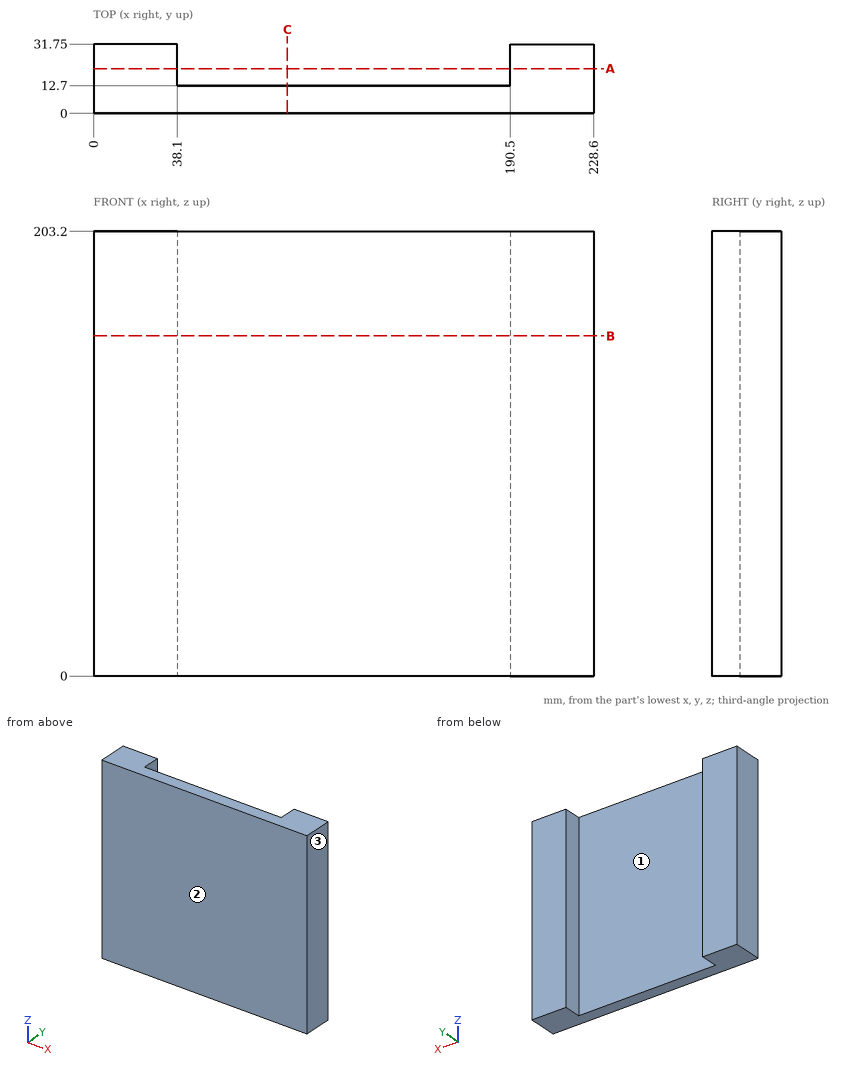
Input: dimensioned drawing with shaded views. Units: mm. Origin: part minimum x, y, z. Coordinates: 2 decimals unless noted, no trailing zeros. Order: outer loops, then holes, each group sorted by start corner. A loop starts at its lowest first (then second) coordinate and runs counter-clockwise, first axis right, second up. Notation, with made-up numbers: (55.5, -14) - (87.5, -14) arc R3 cw to (87.5, -10) - close; hole circle Ø8 at (75.5, 74). An arc over 180 degrees is marked (long way). Return JSON: item names as keys, results as strings. Group by question number.
1. Cut plane B-B (z = 155.5). Output: boundary loops of the cut face in (x, y), plus the area to 3 significant figures.
2. Cut plane C-C (x = 88.5). Output: boundary loops of the cut face in (y, z), plus the area to 3 significant figures.
3. Cut plane A-A (y = 20.5). Output: boundary loops of the cut face in (x, z).
4. Pull-direction query (X, two-part tool) for the marked faces 1, 2 and 3; classes: pulls with the +X half, pulls with the -X half, needs draft (parallel to the pull), parting line crosses it, or undercut.
5. Material intervals for line 1 along X through (y, z) = (19.5, 111.5); line 2 along Y through (x, z) = (190, 52), sorted ascending. Write a range as [from, to].
Resolved:
{
 "1": {"outline": "(0, 0) - (228.6, 0) - (228.6, 31.75) - (190.5, 31.75) - (190.5, 12.7) - (38.1, 12.7) - (38.1, 31.75) - (0, 31.75) - close", "area": "4,350 mm²"},
 "2": {"outline": "(0, 0) - (12.7, 0) - (12.7, 203.2) - (0, 203.2) - close", "area": "2,580 mm²"},
 "3": {"outline": "(0, 0) - (38.1, 0) - (38.1, 203.2) - (0, 203.2) - close; (190.5, 0) - (228.6, 0) - (228.6, 203.2) - (190.5, 203.2) - close"},
 "4": {"face 1": "undercut", "face 2": "needs draft", "face 3": "pulls with the +X half"},
 "5": {"line 1": "x = [0, 38.1], [190.5, 228.6]", "line 2": "y = [0, 12.7]"}
}
